```python
from build123d import *

# Parameters (mm, degrees)
SKETCH2_R                       = 6
BOSS_EXTRUDE1_DEPTH             = 32
BOSS_EXTRUDE2_DEPTH             = 10
CBORE_FOR_M6_SHCS1_D            = 6.4
CBORE_FOR_M6_SHCS1_DEPTH        = 10
CBORE_FOR_M6_SHCS1_CBORE_D      = 10.5
CBORE_FOR_M6_SHCS1_CBORE_DEPTH  = 4
CBORE_FOR_M6_SHCS1_TIP          = 1.922753981
TAP_DRILL_FOR_M6X1_0_TAP1_D     = 5
TAP_DRILL_FOR_M6X1_0_TAP1_DEPTH = 16
TAP_DRILL_FOR_M6X1_0_TAP1_TIP   = 1.502151548
SKETCH2_6_R                     = 6
BOSS_EXTRUDE3_DEPTH             = 10


with BuildPart() as part:
    # Sketch2 → Boss-Extrude1 (new body)
    with BuildSketch(Plane(origin=(0, 0, 0), x_dir=(0, 0, -1), z_dir=(1, 0, 0))):
        with BuildLine():
            Line((-8, 0), (8, 0))
            Line((8, 0), (8, 9))
            Line((8, 9), (32, 9))
            Line((32, 9), (32, 19))
            Line((32, 19), (24.228334067, 19))
            ThreePointArc((24.228334067, 19), (22.616435242, 19.469825663), (21.509410706, 20.732145215))
            Line((21.509410706, 20.732145215), (14.500924593, 35.761892188))
            ThreePointArc((14.500924593, 35.761892188), (0, 45), (-14.500924593, 35.761892188))
            Line((-14.500924593, 35.761892188), (-21.509410706, 20.732145215))
            ThreePointArc((-21.509410706, 20.732145215), (-22.616435242, 19.469825663), (-24.228334067, 19))
            Line((-24.228334067, 19), (-32, 19))
            Line((-32, 19), (-32, 9))
            Line((-32, 9), (-8, 9))
            Line((-8, 9), (-8, 0))
        make_face()
        with Locations((0, 31)):
            Circle(SKETCH2_R, mode=Mode.SUBTRACT)
    extrude(amount=BOSS_EXTRUDE1_DEPTH)

    # Sketch2_5 → Boss-Extrude2 (add)
    with BuildSketch(Plane(origin=(0, 0, 0), x_dir=(0, 0, -1), z_dir=(1, 0, 0))):
        with BuildLine():
            Line((-32, 45), (-32, 19))
            Line((-32, 19), (-24.228334067, 19))
            ThreePointArc((-24.228334067, 19), (-22.616435242, 19.469825663), (-21.509410706, 20.732145215))
            Line((-21.509410706, 20.732145215), (-14.500924593, 35.761892188))
            ThreePointArc((-14.500924593, 35.761892188), (-8.596793734, 42.494263133), (0, 45))
            Line((0, 45), (-32, 45))
        make_face()
        with BuildLine():
            Line((24.228334067, 19), (32, 19))
            Line((32, 19), (32, 45))
            Line((32, 45), (0, 45))
            ThreePointArc((0, 45), (8.596793734, 42.494263133), (14.500924593, 35.761892188))
            Line((14.500924593, 35.761892188), (21.509410706, 20.732145215))
            ThreePointArc((21.509410706, 20.732145215), (22.616435242, 19.469825663), (24.228334067, 19))
        make_face()
    extrude(amount=BOSS_EXTRUDE2_DEPTH)

    # CBORE for M6 SHCS1
    with Locations(Plane(origin=(20, 45, 0), x_dir=(0, 0, 1), z_dir=(0, 1, 0))):
        with Locations((0, 0)):
            CounterBoreHole(CBORE_FOR_M6_SHCS1_D / 2, CBORE_FOR_M6_SHCS1_CBORE_D / 2, CBORE_FOR_M6_SHCS1_CBORE_DEPTH, depth=CBORE_FOR_M6_SHCS1_DEPTH)
            with Locations((0, 0, -(CBORE_FOR_M6_SHCS1_DEPTH + CBORE_FOR_M6_SHCS1_TIP / 2))):  # 118° drill point
                Cone(0, CBORE_FOR_M6_SHCS1_D / 2, CBORE_FOR_M6_SHCS1_TIP, mode=Mode.SUBTRACT)

    # Tap Drill for M6x1.0 Tap1
    with Locations(Plane(origin=(0, 0, 0), x_dir=(-1, 0, 0), z_dir=(0, -1, 0))):
        with Locations((-24, 0), (-8, 0)):
            Hole(TAP_DRILL_FOR_M6X1_0_TAP1_D / 2, depth=TAP_DRILL_FOR_M6X1_0_TAP1_DEPTH)
            with Locations((0, 0, -(TAP_DRILL_FOR_M6X1_0_TAP1_DEPTH + TAP_DRILL_FOR_M6X1_0_TAP1_TIP / 2))):  # 118° drill point
                Cone(0, TAP_DRILL_FOR_M6X1_0_TAP1_D / 2, TAP_DRILL_FOR_M6X1_0_TAP1_TIP, mode=Mode.SUBTRACT)

    # Sketch2_6 → Boss-Extrude3 (add)
    with BuildSketch(Plane(origin=(0, 0, 0), x_dir=(0, 0, -1), z_dir=(1, 0, 0))):
        with Locations((0, 31)):
            Circle(SKETCH2_6_R)
    extrude(amount=BOSS_EXTRUDE3_DEPTH)


solid = part.part
```
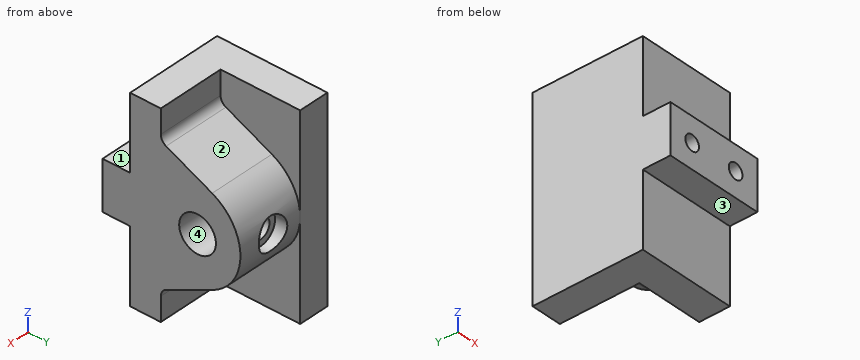
Here's how the part is built. I have some questions about the finished solid (model axes, mm). Face numbers are marked on the shaded views. A direction names the side the tool comes from. Round coordinates to 2 decimals unless told otherwise and drop trailing zeros. Write each loop counter-clockwise with the first axis right and the second up, starting at its lowest first coordinate (ties: lowest second). Pieces come first, ordered by that corner, then holes. Notation, with made-up numbers: M 25,-2.5 L 43,-2.5 A12 cw 43,13.5 Z; hole C 67.25,10.5 d10. An arc over 180 degrees is marked long. Answer as CSV lines item,"result". Start each with the question number.
1. Suppose I cut it at C-C on z = 18.5. Write out the boundary of the cut face in (x, y), then the cut area to 3 significant figures.
2. On a 3-axis mill with a long thin cutter (end or side, diameter ignored), from which of +Z, -Z, +X, -X, +Y, -Y can I reach the whole of each face in a straight line? I mean the marked faces 1, 2, 3 and 4. Say none if no direction works.
3. I'm going to push flat-ended pins straight in: pin 1 Ø5 at (x, z) = (14, -22.5) entering from -Y; pin 2 Ø4 at (x, z) = (21.5, -29.5) entering from +Y; pin 3 Ø7 at (x, y) = (16, 4.5) entering from +Z. Where does each tip first touch, or does it pass through?
4. Suppose I cut it at B-B on x = 4. Write out the boundary of the cut face in (y, z).
5. Suppose I cut it at D-D on y = 32.5. Write out the boundary of the cut face in (x, z), then the cut area to 3 significant figures.
6. I need wall thicknesses on probe 1 along Z at (x, y) = (24, 12); probe 2 along Y at (x, z) = (7, 8.5); probe 3 along X at (y, z) = (38.5, -20.5). Which ranges of each line are inside material? Lowest first, please.
7. Suppose I cut it at A-A on y = 5.5. Write out the boundary of the cut face in (x, z), then the cut area to 3 significant figures.
Check result:
1,outline,"M 0,9 L 32,9 L 32,27.19 L 10,27.19 L 10,45 L 0,45 Z"
1,area,"760 mm2"
2,face 1,"+Z, +X, -X, -Y"
2,face 2,"+Z, +X, +Y"
2,face 3,"-Z, +X, -X, -Y"
2,face 4,"+X"
3,pin 1,"stops at y = 9"
3,pin 2,"stops at y = 19"
3,pin 3,"stops at z = 8"
4,outline,"M 0,-8 L 9,-8 L 9,-32 L 45,-32 L 45,32 L 9,32 L 9,8 L 0,8 Z"
5,outline,"M 0,-32 L 10,-32 L 10,-16.02 L 32,-16.02 L 32,-5.81 L 10,-5.81 L 10,5.81 L 32,5.81 L 32,16.02 L 10,16.02 L 10,32 L 0,32 Z"
5,area,"1,090 mm2"
6,probe 1,"z = -32 to -2.5, 2.5 to 32"
6,probe 2,"y = 9 to 45"
6,probe 3,"x = 0 to 10"
7,outline,"M 0,-8 L 32,-8 L 32,8 L 0,8 Z; hole C 8,0 d5; hole C 24,0 d5"
7,area,"473 mm2"
